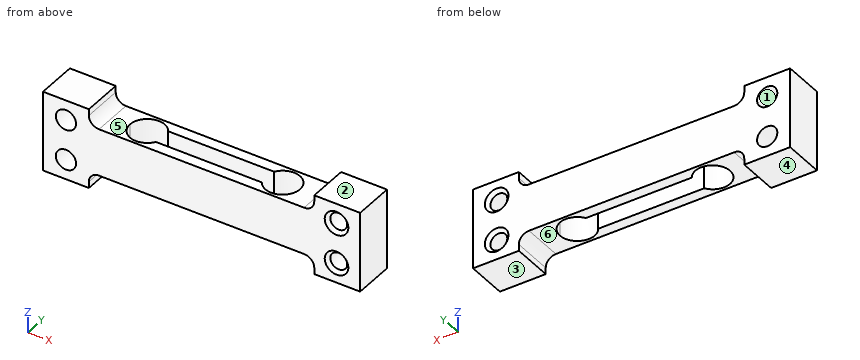
```python
from build123d import *

# Parameters (mm, degrees)
BOSS_EXTRUDE1_DEPTH        = 3
CUT_EXTRUDE1_DEPTH         = 26.505930683
M3_TAPPED_HOLE1_AT_2_COUNT = 2
M3_TAPPED_HOLE1_AT_2_PITCH = 6
SKETCH6_R                  = 1.5
CUT_EXTRUDE2_DEPTH         = 25.973035458


with BuildPart() as part:
    # Sketch1 → Boss-Extrude1 (new, symmetric)
    with BuildSketch(Plane(origin=(0, 0, 0), x_dir=(1, 0, 0), z_dir=(0, 1, 0))):
        with BuildLine():
            Line((0, -3.5), (0, 3.5))
            Line((0, 3.5), (15.2, 3.5))
            ThreePointArc((15.2, 3.5), (16.260660172, 3.939339828), (16.7, 5))
            Line((16.7, 5), (16.7, 5.95))
            Line((16.7, 5.95), (23.5, 5.95))
            Line((23.5, 5.95), (23.5, -5.95))
            Line((23.5, -5.95), (16.7, -5.95))
            Line((16.7, -5.95), (16.7, -5))
            ThreePointArc((16.7, -5), (16.260660172, -3.939339828), (15.2, -3.5))
            Line((15.2, -3.5), (0, -3.5))
        make_face()
    extrude(amount=BOSS_EXTRUDE1_DEPTH, both=True)

    # Sketch2 → Cut-Extrude1 (cut, through all)
    with BuildSketch(Plane.XY.offset(3.5)):
        with BuildLine():
            ThreePointArc((7.847845894, 1.375), (7.45, 0), (7.847845894, -1.375))
            Line((7.847845894, -1.375), (10.025, -1.375))
            Line((10.025, -1.375), (10.025, 1.375))
            Line((10.025, 1.375), (7.847845894, 1.375))
        make_face()
        with BuildLine():
            Line((10.025, -1.375), (7.847845894, -1.375))
            ThreePointArc((7.847845894, -1.375), (10.740700069, -2.473539652), (12.6, 0))
            ThreePointArc((12.6, 0), (10.740700069, 2.473539652), (7.847845894, 1.375))
            Line((7.847845894, 1.375), (10.025, 1.375))
            Line((10.025, 1.375), (10.025, -1.375))
        make_face()
        with BuildLine():
            Line((0, 1.375), (0, -1.375))
            Line((0, -1.375), (7.847845894, -1.375))
            ThreePointArc((7.847845894, -1.375), (7.45, 0), (7.847845894, 1.375))
            Line((7.847845894, 1.375), (0, 1.375))
        make_face()
    extrude(amount=-CUT_EXTRUDE1_DEPTH, mode=Mode.SUBTRACT)

    # Mirror1: part across plane


with BuildPart() as part_1:
    add(part.part)
    add(part.part.mirror(Plane(origin=(0, 0, 0), x_dir=(0, 0, 1), z_dir=(1, 0, 0))))

    # Sketch5 → M3 Tapped Hole1 (revolve, cut)
    with BuildSketch(Plane(origin=(20, 3, -3), x_dir=(0, 0, 1), z_dir=(1, 0, 0))):
        Polygon((0, 0), (0, 6), (1.75, 6), (1.25, 5.5), (1.25, 0.5), (1.75, 0), align=None)
    m3_tapped_hole1 = revolve(axis=Axis((20, 9.35, -3), (0, -1, 0)), mode=Mode.SUBTRACT)

    # M3 Tapped Hole1 at 2: M3 Tapped Hole1 ×2
    with Locations(*[(0, 0, i * M3_TAPPED_HOLE1_AT_2_PITCH) for i in range(1, M3_TAPPED_HOLE1_AT_2_COUNT)]):
        add(m3_tapped_hole1, mode=Mode.SUBTRACT)

    # Sketch6 → Cut-Extrude2 (cut, through all)
    with BuildSketch(Plane(origin=(0, 3, 0), x_dir=(1, 0, 0), z_dir=(0, 1, 0))):
        with Locations(Location((-20.1, 3, 0), (0, 0, 270))):
            Circle(SKETCH6_R)
        with Locations(Location((-20.1, -3, 0), (0, 0, 270))):
            Circle(SKETCH6_R)
    extrude(amount=-CUT_EXTRUDE2_DEPTH, mode=Mode.SUBTRACT)


solid = part_1.part
```
Geometry: final body of the model. Coordinates: model frame, mm. Face numbers are marked on the shaded views. A direction names the side the tool comes from. Round coordinates to 2 decimals unless told otherwise and drop trailing zeros. Order: outer loops, then holes, each group sorted by start corner. A loop starts at its lowest first (then second) coordinate and runs counter-clockwise, first axis right, second up. Notation, with made-up numbers: (64.5, 38.5) - (97.5, 38.5) arc R18 cw to (97.5, 64.5) - close; hole circle Ø2 at (89, 18.25). An arc over 180 degrees is marked (long way). Use CSV: the item, a comma, the result in double quotes. Start each with the question number.
Q1. Section query C-C (y = -1.85). Return loops of the section in (x, z).
Q2. Section query B-B (z = 3). Return loops of the section in (x, y) (3 decimals).
Q3. Mould query, pull axis Z, two halves, no side actions, for the marked faces 1, 2 and 3. Classes: +Z half, -Z half, draft (parallel to the pull), parting line (faces both ways), or undercut.
Q4. Material intervals for line 1 along Z through (x, y) = (20, -0.55); line 2 along Y through (x, z) = (2.5, 1.25) (3 decimals); line 3 along X through (y, z) = (0.25, -3), sorted ascending. Write a range as from..to.
Q5. Access query for the marked faces 4, 5 and 6. Directions: +Z, -Z, +X, -X, +Y, -Y. A direction counts if a zero-diameter tool reaches every point of the face in a straight line with its end or side. Return the directions, or none.
Q6. Section query A-A (x = -20.1). Return loops of the section in (y, z), and give its area (3 significant figures).
Q7. First-contact query: pin 1 (3 mm diameter, centred on x = -2, y = 0, fed in from -Z); pin 2 (5 mm diameter, centred on x = -20.1, z = -3, fed in from +Y); pin 3 (3 mm diameter, centred on x = -13, y = 0, fed in from +Z); pin 4 (3 mm diameter, centred on x = 20, z = 3, fed in from +Y). Flat tips, straight axial feed; report the tip coordinate or a pass-through.
Q8. Section query D-D (x = 6). Return loops of the section in (y, z) (3 decimals), and give its area (4 significant figures).
Result set:
1,outline,"(-23.5, -5.95) - (-16.7, -5.95) - (-16.7, -5) arc R1.5 cw to (-15.2, -3.5) - (-11.82, -3.5) - (-11.82, 3.5) - (-15.2, 3.5) arc R1.5 cw to (-16.7, 5) - (-16.7, 5.95) - (-23.5, 5.95) - close; (-8.23, -3.5) - (8.23, -3.5) - (8.23, 3.5) - (-8.23, 3.5) - close; (11.82, -3.5) - (15.2, -3.5) arc R1.5 cw to (16.7, -5) - (16.7, -5.95) - (23.5, -5.95) - (23.5, 5.95) - (16.7, 5.95) - (16.7, 5) arc R1.5 cw to (15.2, 3.5) - (11.82, 3.5) - close; hole circle Ø3 at (-20.1, -3); hole circle Ø3 at (-20.1, 3); hole circle Ø2.5 at (20, -3); hole circle Ø2.5 at (20, 3)"
2,outline,"(-23.5, -3) - (-21.6, -3) - (-21.6, 3) - (-23.5, 3) - close; (-18.6, -3) - (18.25, -3) - (18.75, -2.5) - (18.75, 2.5) - (18.25, 3) - (-18.6, 3) - close; (21.25, -2.5) - (21.75, -3) - (23.5, -3) - (23.5, 3) - (21.75, 3) - (21.25, 2.5) - close; hole (-7.848, -1.375) - (7.848, -1.375) arc R2.575 ccw (long way) to (7.848, 1.375) - (-7.848, 1.375) arc R2.575 ccw (long way) to start"
3,face 1,"undercut"
3,face 2,"+Z half"
3,face 3,"-Z half"
4,line 1,"z = -5.95..-4.25, -1.75..1.75, 4.25..5.95"
4,line 2,"y = -3..-1.375, 1.375..3"
4,line 3,"x = -23.5..-21.6, -18.6..-12.59, 12.59..18.75, 21.25..23.5"
5,face 4,"-Z, +X, -X, +Y, -Y"
5,face 5,"+Z, +Y, -Y"
5,face 6,"-Z, +Y, -Y"
6,outline,"(-3, -5.95) - (3, -5.95) - (3, -4.5) - (-3, -4.5) - close; (-3, -1.5) - (3, -1.5) - (3, 1.5) - (-3, 1.5) - close; (-3, 4.5) - (3, 4.5) - (3, 5.95) - (-3, 5.95) - close"
6,area,"35.4 mm2"
7,pin 1,"stops at z = -3.5"
7,pin 2,"stops at y = 3"
7,pin 3,"stops at z = 3.5"
7,pin 4,"stops at y = 2.75"
8,outline,"(-3, -3.5) - (-1.375, -3.5) - (-1.375, 3.5) - (-3, 3.5) - close; (1.375, -3.5) - (3, -3.5) - (3, 3.5) - (1.375, 3.5) - close"
8,area,"22.75 mm2"
